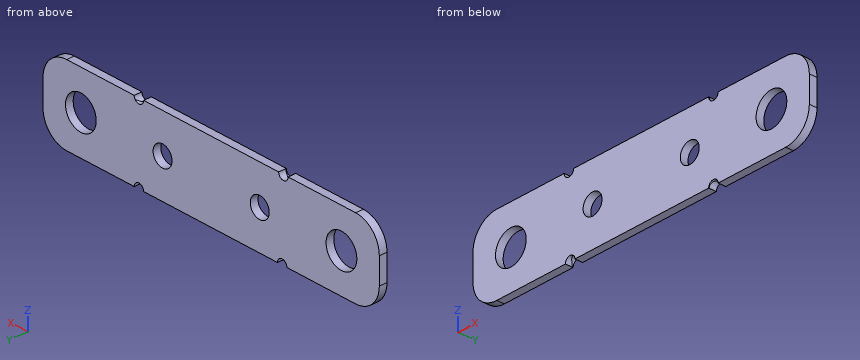
from build123d import *

# Parameters (mm, degrees)
SM_BASE_FLANGE_2_DEPTH      = 15
SKETCH_26_R                 = 3.25
CUT_EXTRUDE_1_DEPTH         = 42.400483089
FILLET_1_R                  = 5
CUT_EXTRUDE_2_OUTLINE_W     = 33
CUT_EXTRUDE_2_OUTLINE_H     = 15
CUT_EXTRUDE_2_OUTLINE_R     = 2
CUT_EXTRUDE_2_DEPTH         = 20
CUT_EXTRUDE_START           = -1.5
CUT_EXTRUDE_2_2_OUTLINE_R   = 2
CUT_EXTRUDE_2_2_DEPTH       = 1.5
CUT_EXTRUDE_2_3_OUTLINE_R   = 2
CUT_EXTRUDE_2_3_OUTLINE_R_2 = 3.25
CUT_EXTRUDE_2_3_DEPTH       = 1.5


# Read off the part's stored shape, not the designer's step: Вырез-Вытянуть2
# Sheet-metal steps are written as plain solids
with BuildPart() as part:
    # Эскиз1 → Базовая кромка2 (new body)
    with BuildSketch(Plane.XY):
        with BuildLine():
            Line((0, 20), (0, 1.5))
            ThreePointArc((0, 1.5), (0.439339828, 0.439339828), (1.5, 0))
            Line((1.5, 0), (28.5, 0))
            ThreePointArc((28.5, 0), (29.560660172, 0.439339828), (30, 1.5))
            Line((30, 1.5), (30, 20))
            Line((30, 20), (31.5, 20))
            Line((31.5, 20), (31.5, 1.5))
            ThreePointArc((31.5, 1.5), (30.621320344, -0.621320344), (28.5, -1.5))
            Line((28.5, -1.5), (1.5, -1.5))
            ThreePointArc((1.5, -1.5), (-0.621320344, -0.621320344), (-1.5, 1.5))
            Line((-1.5, 1.5), (-1.5, 20))
            Line((-1.5, 20), (0, 20))
        make_face()
    extrude(amount=SM_BASE_FLANGE_2_DEPTH)

    # Эскиз26 → Вырез-Вытянуть1 (cut, through all)
    with BuildSketch(Plane(origin=(31.5, 0, 0), x_dir=(0, 0, -1), z_dir=(1, 0, 0))):
        with Locations((-7.5, 12)):
            Circle(SKETCH_26_R)
    extrude(amount=-CUT_EXTRUDE_1_DEPTH, mode=Mode.SUBTRACT)

    # Скругление1
    fillet_1_edges = [part.edges().sort_by_distance(p)[0] for p in [
        (-0.75, 20, 0),
        (30.75, 20, 0),
        (-0.75, 20, 15),
        (30.75, 20, 15),
    ]]
    fillet(fillet_1_edges, radius=FILLET_1_R)

    # Вырез-Вытянуть2 outline → Вырез-Вытянуть2 (cut)
    with BuildSketch(Plane(origin=(0, 0, 0), x_dir=(1, 0, 0), z_dir=(0, 1, 0))):
        with Locations((15, -7.5)):
            Rectangle(CUT_EXTRUDE_2_OUTLINE_W, CUT_EXTRUDE_2_OUTLINE_H)
        with Locations((25.267145868, -7.5)):
            Circle(CUT_EXTRUDE_2_OUTLINE_R, mode=Mode.SUBTRACT)
        with Locations((4.732854132, -7.5)):
            Circle(CUT_EXTRUDE_2_OUTLINE_R, mode=Mode.SUBTRACT)
    extrude(amount=CUT_EXTRUDE_2_DEPTH, mode=Mode.SUBTRACT)

    # Cut-Extrude 2 2 outline → Cut-Extrude 2 2 (cut)
    with BuildSketch(Plane(origin=(0, 0, 0), x_dir=(1, 0, 0), z_dir=(0, 1, 0)).offset(CUT_EXTRUDE_START)):
        with BuildLine():
            ThreePointArc((31.267145868, -15), (30.267145868, -14), (29.267145868, -15))
            Line((29.267145868, -15), (31.267145868, -15))
        make_face()
        with BuildLine():
            Line((31.267145868, 0), (29.267145868, 0))
            ThreePointArc((29.267145868, 0), (30.267145868, -1), (31.267145868, 0))
        make_face()
        with BuildLine():
            ThreePointArc((0.732854132, -15), (-0.267145868, -14), (-1.267145868, -15))
            Line((-1.267145868, -15), (0.732854132, -15))
        make_face()
        with BuildLine():
            Line((1, 0), (-1, 0))
            ThreePointArc((-1, 0), (0, -1), (1, 0))
        make_face()
        with Locations((25.267145868, -7.5)):
            Circle(CUT_EXTRUDE_2_2_OUTLINE_R)
        with Locations((4.732854132, -7.5)):
            Circle(CUT_EXTRUDE_2_2_OUTLINE_R)
    extrude(amount=CUT_EXTRUDE_2_2_DEPTH, mode=Mode.SUBTRACT)

    # Cut-Extrude 2 3 outline → Cut-Extrude 2 3 (add)
    with BuildSketch(Plane(origin=(0, 0, 0), x_dir=(1, 0, 0), z_dir=(0, 1, 0)).offset(CUT_EXTRUDE_START)):
        with BuildLine():
            Line((31.267145868, -15), (45.534291735, -15))
            ThreePointArc((45.534291735, -15), (49.069825641, -13.535533906), (50.534291735, -10))
            Line((50.534291735, -10), (50.534291735, -5))
            ThreePointArc((50.534291735, -5), (49.069825641, -1.464466094), (45.534291735, 0))
            Line((45.534291735, 0), (31.267145868, 0))
            ThreePointArc((31.267145868, 0), (30.267145868, -1), (29.267145868, 0))
            Line((29.267145868, 0), (1, 0))
            ThreePointArc((1, 0), (0, -1), (-1, 0))
            Line((-1, 0), (-15.534291735, 0))
            ThreePointArc((-15.534291735, 0), (-19.069825641, -1.464466094), (-20.534291735, -5))
            Line((-20.534291735, -5), (-20.534291735, -10))
            ThreePointArc((-20.534291735, -10), (-19.069825641, -13.535533906), (-15.534291735, -15))
            Line((-15.534291735, -15), (-1.267145868, -15))
            ThreePointArc((-1.267145868, -15), (-0.267145868, -14), (0.732854132, -15))
            Line((0.732854132, -15), (29.267145868, -15))
            ThreePointArc((29.267145868, -15), (30.267145868, -14), (31.267145868, -15))
        make_face()
        with Locations((25.267145868, -7.5)):
            Circle(CUT_EXTRUDE_2_3_OUTLINE_R, mode=Mode.SUBTRACT)
        with Locations((4.732854132, -7.5)):
            Circle(CUT_EXTRUDE_2_3_OUTLINE_R, mode=Mode.SUBTRACT)
        with Locations((42.534291735, -7.5)):
            Circle(CUT_EXTRUDE_2_3_OUTLINE_R_2, mode=Mode.SUBTRACT)
        with Locations((-12.534291735, -7.5)):
            Circle(CUT_EXTRUDE_2_3_OUTLINE_R_2, mode=Mode.SUBTRACT)
    extrude(amount=CUT_EXTRUDE_2_3_DEPTH)


solid = part.part
Could you check a few things on this model? Use its own coordinates, in mm. Round coordinates to 2 decimals unless told otherwise and drop trailing zeros. Write each loop counter-clockwise with the first axis right and the second up, starting at its lowest first coordinate (ties: lowest second). Pieces come first, ordered by that corner, then holes. Notation, with made-up numbers: (-19, 63) - (20, 63) arc R11 cw to (20, 78) - close; hole circle Ø8 at (-37.75, -39.75). An arc over 180 degrees is marked (long way). Use a Markdown table: item, result.
Q1. Please list where these lines run through material, in increasing order: L1, parallel to X at y = -0.9, z = 7.5; L2, parallel to X at y = -1.4, z = 10.5; L3, parallel to Z at x = 27, y = -0.25.
Output values:
| item | result |
|---|---|
| L1 | -20.53 to -15.78, -9.28 to 2.73, 6.73 to 23.27, 27.27 to 39.28, 45.78 to 50.53 |
| L2 | -20.51 to -13.78, -11.28 to 41.28, 43.78 to 50.51 |
| L3 | 0 to 6.5, 8.5 to 15 |
Q2. For pin 1 (3 mm diameter, centred on x = 25.27, z = 7.5, fed in from +Y), with a flat end and sliding along its axis, tell me the tip position at first contact or that it passes through.
Output values:
| item | result |
|---|---|
| pin 1 | through |
Q3. I want a section at A-A (y = -0.55). List the corners of the cut face in (x, z) for me.
Output values:
| item | result |
|---|---|
| outline | (-20.53, 5) arc R5 ccw to (-15.53, 0) - (-1, 0) arc R1 cw to (1, 0) - (29.27, 0) arc R1 cw to (31.27, 0) - (45.53, 0) arc R5 ccw to (50.53, 5) - (50.53, 10) arc R5 ccw to (45.53, 15) - (31.27, 15) arc R1 cw to (29.27, 15) - (0.73, 15) arc R1 cw to (-1.27, 15) - (-15.53, 15) arc R5 ccw to (-20.53, 10) - close; hole circle Ø6.5 at (-12.53, 7.5); hole circle Ø4 at (4.73, 7.5); hole circle Ø4 at (25.27, 7.5); hole circle Ø6.5 at (42.53, 7.5) |
Q4. I want a section at B-B (x = 4.5). List the corners of the cut face in (y, z) for me.
Output values:
| item | result |
|---|---|
| outline | (-1.5, 0) - (0, 0) - (0, 5.51) - (-1.5, 5.51) - close; (-1.5, 9.49) - (0, 9.49) - (0, 15) - (-1.5, 15) - close |
